Can you work these out from the model? Positions are in its coordinate system, mm. A direction names the side the tool comes from. Give positions to 0.01 mm unless a question says otherwise; leave off trailing zeros. Write each loop counter-clockwise with the first axis right and the second up, starting at its lowest first coordinate (ties: lowest second). Pieces come first, ordered by that corner, then holes.
```python
from build123d import *

# Parameters (mm, degrees)
FILLET_1_R          = 1
SKETCH_2_R          = 4.5
SKETCH_2_R_2        = 3.75
CUT_EXTRUDE_1_DEPTH = 0.2


with BuildPart() as part:
    # 草图1 → 旋转1 (revolve)
    with BuildSketch(Plane.XY, mode=Mode.PRIVATE) as revolve_1_sk:
        Polygon((0, 0), (7, 0), (7, -1.5), (6, -1.5), (6, -21.5), (0, -21.5), align=None)
    revolve(revolve_1_sk.sketch.rotate(Axis((0, 0, 0), (0, 1, 0)), 90), axis=Axis((0, 0, 0), (0, 1, 0)))

    # 圆角1
    fillet_1_edges = [part.edges().sort_by_distance(p)[0] for p in [
        (0, 0, 7),
    ]]
    fillet(fillet_1_edges, radius=FILLET_1_R)

    # 草图2 → 切除-拉伸1 (cut)
    with BuildSketch(Plane(origin=(0, 0, 0), x_dir=(1, 0, 0), z_dir=(0, 1, 0))):
        with Locations(Location((0, 0, 0), (0, 0, 270))):
            Circle(SKETCH_2_R)
        with Locations(Location((0, 0, 0), (0, 0, 270))):
            Circle(SKETCH_2_R_2, mode=Mode.SUBTRACT)
    extrude(amount=-CUT_EXTRUDE_1_DEPTH, mode=Mode.SUBTRACT)


solid = part.part
```
1) Please list where these lines run through material, in increasing order: L1, parallel to Y at x = 3, z = -5.25; L2, parallel to Y at x = -3.75, z = 1.5; L3, parallel to X at y = -10.5, z = 0.
Values follow:
L1: y = -1.5 to 0
L2: y = -21.5 to -0.2
L3: x = -6 to 6
2) For pin 1 Ø2 at (y, z) = (-10, 3.5) entering from +X; pin 2 Ø2 at (x, y) = (1.5, -18) entering from +Z; pin 3 Ø5 at (y, z) = (-6, 2.5) entering from -X, each with a flat end and sliding along its axis, tell me the tip position at first contact or that it passes through.
Values follow:
pin 1: stops at x = 5.45
pin 2: stops at z = 5.98
pin 3: stops at x = -6
3) Suppose I cut it at A-A on z = 0. Write out the boundary of the cut face in (x, y).
Values follow:
outline: (-7, -1.5) - (-6, -1.5) - (-6, -21.5) - (6, -21.5) - (6, -1.5) - (7, -1.5) - (7, -1) arc R1 ccw to (6, 0) - (4.5, 0) - (4.5, -0.2) - (3.75, -0.2) - (3.75, 0) - (-3.75, 0) - (-3.75, -0.2) - (-4.5, -0.2) - (-4.5, 0) - (-6, 0) arc R1 ccw to (-7, -1) - close
4) Suppose I cut it at C-C on y = -11.25. Write out the boundary of the cut face in (x, z), plus the area to 3 significant figures.
Values follow:
outline: circle Ø12 at (0, 0)
area: 113 mm2
5) For faces 4 (the face through (-2, -1.5, -6)), 5 (the face through (6.21, -1.25, -3.23)), which set-ups out of +Z, -Z, +X, -X, +Y, -Y let a thin tool reach every point of the face, with its end or its side?
Values follow:
face 4: -Y
face 5: +Y, -Y
6) If we mould it in two halves opening along X, with no side actions, what happens to faces 1 (the face through (4, -0.2, -1)), 2 (the face through (-1.802, -11.64, -5.723)), 3 (the face through (0, -21.5, 0))? For each: +X half, -X half, draft (parallel to the pull), parting line (faces both ways), or undercut.
Values follow:
face 1: undercut
face 2: parting line
face 3: draft
7) Suppose I cut it at B-B on x = 0. Write out the boundary of the cut face in (y, z).
Values follow:
outline: (-21.5, -6) - (-1.5, -6) - (-1.5, -7) - (-1, -7) arc R1 ccw to (0, -6) - (0, -4.5) - (-0.2, -4.5) - (-0.2, -3.75) - (0, -3.75) - (0, 3.75) - (-0.2, 3.75) - (-0.2, 4.5) - (0, 4.5) - (0, 6) arc R1 ccw to (-1, 7) - (-1.5, 7) - (-1.5, 6) - (-21.5, 6) - close
